Geometry: final body of the model. Coordinates: model frame, mm. Face numbers are marked on the shaded views. A direction names the side the tool comes from. Round coordinates to 2 decimals unless told otherwise and drop trailing zeros. Write each loop counter-clockwise with the first axis right and the second up, starting at its lowest first coordinate (ties: lowest second). Pieces come first, ordered by that corner, then holes. Notation, with made-up numbers: (-20.75, 7) - (-11.75, 7) arc R30 ccw to (-11.75, 37) - close; hole circle Ø6 at (26, 74). An arc over 180 degrees is marked (long way). Write each question's results on one line, items separated by ' | '.
from build123d import *

# Parameters (mm, degrees)
EXTRUDE_1_DEPTH     = 40
CUT_EXTRUDE_1_REACH = 122
SKETCH_5_R          = 13
SKETCH_6_R          = 3.25
CUT_EXTRUDE_2_DEPTH = 20


with BuildPart() as part:
    # 草图1 → 凸台-拉伸1 (new body)
    with BuildSketch(Plane(origin=(0, 0, 0), x_dir=(0, 0, -1), z_dir=(1, 0, 0))):
        with BuildLine():
            Line((0, 0), (77, 0))
            ThreePointArc((77, 0), (82.656854249, 2.343145751), (85, 8))
            Line((85, 8), (85, 112))
            ThreePointArc((85, 112), (82.656854249, 117.656854249), (77, 120))
            Line((77, 120), (0, 120))
            Line((0, 120), (0, 110))
            Line((0, 110), (67, 110))
            ThreePointArc((67, 110), (72.656854249, 107.656854249), (75, 102))
            Line((75, 102), (75, 18))
            ThreePointArc((75, 18), (72.656854249, 12.343145751), (67, 10))
            Line((67, 10), (0, 10))
            Line((0, 10), (0, 0))
        make_face()
    extrude(amount=EXTRUDE_1_DEPTH)

    # 草图5 → 切除-拉伸1 (cut, up to next)
    with BuildSketch(Plane.XZ, mode=Mode.PRIVATE) as cut_extrude_1_sk1:
        with Locations((20, -35)):
            Circle(SKETCH_5_R)
    cut_extrude_1_tool1 = extrude(cut_extrude_1_sk1.sketch, amount=-CUT_EXTRUDE_1_REACH, mode=Mode.PRIVATE) & part.part
    add(cut_extrude_1_tool1.solids().sort_by_distance((20, 0, -35))[0], mode=Mode.SUBTRACT)

    # 草图6 → 切除-拉伸2 (cut)
    with BuildSketch(Plane.XZ):
        with Locations((20, -7)):
            Circle(SKETCH_6_R)
        with Locations((20, -63)):
            Circle(SKETCH_6_R)
    extrude(amount=-CUT_EXTRUDE_2_DEPTH, mode=Mode.SUBTRACT)


solid = part.part
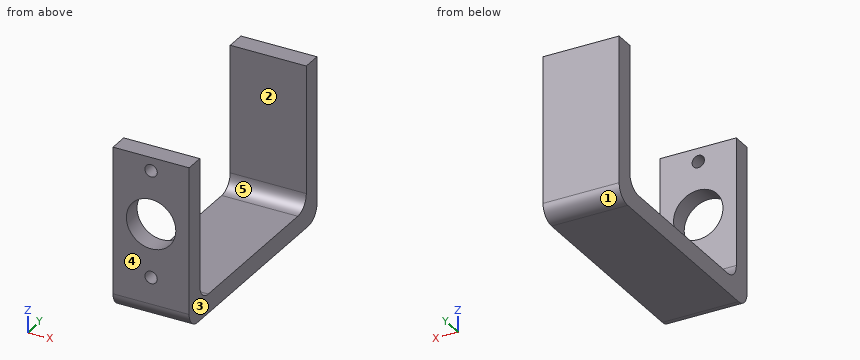
Q1. Pin query (flat end, axial travel): pin 1 (4 mm diameter, centred on x = 20, z = -63, fed in from -Y); pin 2 (4 mm diameter, centred on x = 22.5, y = 85.5, fed in from +Z). Return the tip coordinate at first contact, or that it passes through.
Answer block:
pin 1: y = 110 | pin 2: z = -75
Q2. Mould query, pull axis Y, two halves, no side actions, for the marked faces 1, 2 and 3. Classes: pulls with the +Y half, pulls with the -Y half, needs draft (parallel to the pull), parting line crosses it, or undercut.
Answer block:
face 1: pulls with the +Y half | face 2: undercut | face 3: needs draft
Q3. Section query D-D, the plane x = 4. Return loops of the section in (y, z), plus the area to 3 significant figures.
Answer block:
outline: (0, -77) arc R8 ccw to (8, -85) - (112, -85) arc R8 ccw to (120, -77) - (120, 0) - (110, 0) - (110, -67) arc R8 cw to (102, -75) - (18, -75) arc R8 cw to (10, -67) - (10, 0) - (0, 0) - close | area: 2,700 mm2
Q4. Section query C-C, the plane z = -35. Return loops of the section in (x, y).
Answer block:
outline: (0, 0) - (7, 0) - (7, 10) - (0, 10) - close; (0, 110) - (40, 110) - (40, 120) - (0, 120) - close; (33, 0) - (40, 0) - (40, 10) - (33, 10) - close
Q5. Section query A-A, the plane x = 25. Return loops of the section in (y, z).
Answer block:
outline: (0, -77) arc R8 ccw to (8, -85) - (112, -85) arc R8 ccw to (120, -77) - (120, 0) - (110, 0) - (110, -67) arc R8 cw to (102, -75) - (18, -75) arc R8 cw to (10, -67) - (10, -47) - (0, -47) - close; (0, -23) - (10, -23) - (10, 0) - (0, 0) - close
Q6. Section query B-B, the plane z = -15.5. Return loops of the section in (x, y).
Answer block:
outline: (0, 0) - (40, 0) - (40, 10) - (0, 10) - close; (0, 110) - (40, 110) - (40, 120) - (0, 120) - close
Q7. Ray query, line 1 along Y through (x, z) = (9, -45.5); line 2 along Z through (x, y) = (20, 4); line 3 along Z through (x, y) = (35, 77.5). Return the intervals inside material, ascending.
Answer block:
line 1: 0 to 10, 110 to 120 | line 2: -83.93 to -66.25, -59.75 to -48, -22 to -10.25, -3.75 to 0 | line 3: -85 to -75
Q8. Access query for the marked faces 4 and 5. Directions: +Z, -Z, +X, -X, +Y, -Y. A direction counts if a zero-diameter tool reaches every point of the face in a straight line with its end or side. Return the directions, or none.
Answer block:
face 4: +Z, -Z, +X, -X, -Y | face 5: +Z, +X, -X
